The drawing under review shows one solid part. Ordinate dimensions are in mm from its lowest x, y, z. A direction names the side the tool comes from. Give positions to 0.01 mm unless a question says otherwise; leave off trailing zeros. Loops run counter-clockwise (first coordinate to the right, second up) from the corner with the lowest first, then second, coordinate; pieces in that order, holes last.
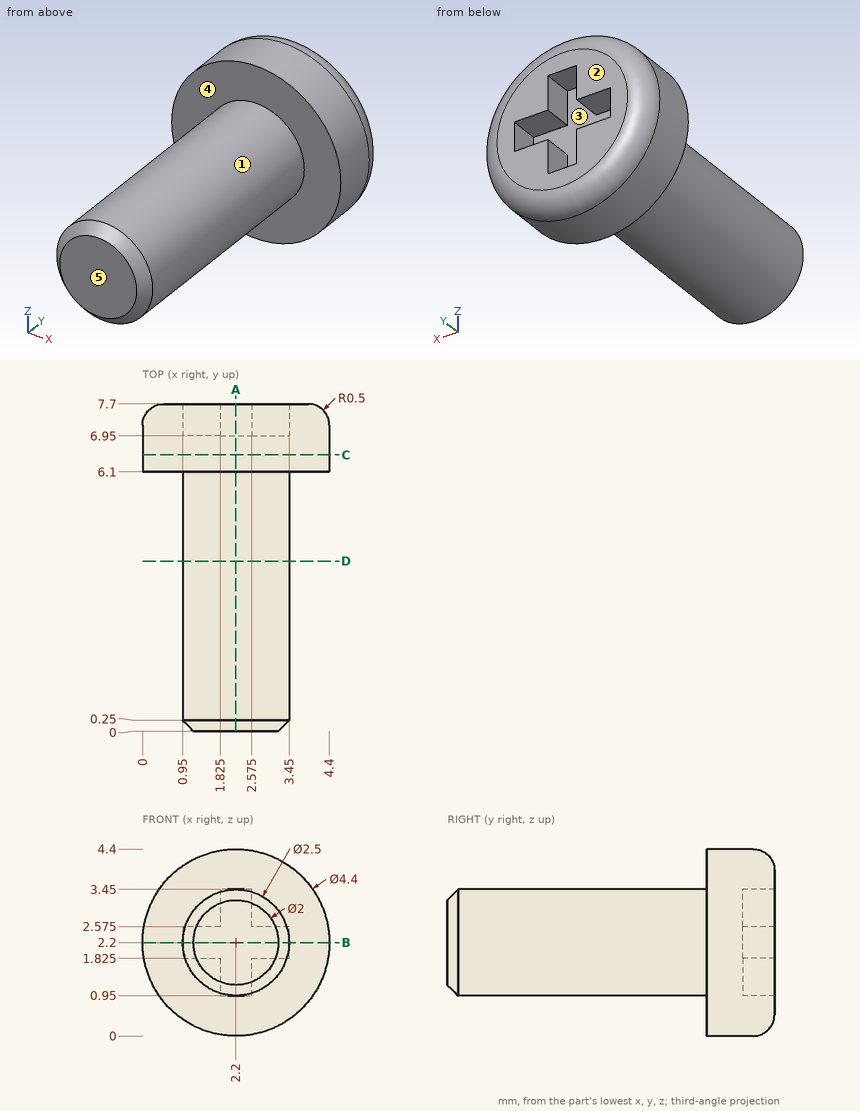
Item 1: Take a section at D-D on y = 4. Give the boundary of the cut face in (x, z).
Answer:
outline: circle Ø2.5 at (2.2, 2.2)
Item 2: Tool access review of the marked faces 4 and 5: name each direction out of +Z, -Z, +X, -X, +Y, -Y from which nothing blocks a thin tool from reaching the whole face with its end or side.
Answer:
face 4: -Y
face 5: +Z, -Z, +X, -X, -Y
Item 3: Take a section at A-A on x = 2.2. Give the boundary of the cut face in (y, z).
Answer:
outline: (0, 1.2) - (0.25, 0.95) - (6.1, 0.95) - (6.1, 0) - (7.2, 0) arc R0.5 ccw to (7.7, 0.5) - (7.7, 0.95) - (6.95, 0.95) - (6.95, 3.45) - (7.7, 3.45) - (7.7, 3.9) arc R0.5 ccw to (7.2, 4.4) - (6.1, 4.4) - (6.1, 3.45) - (0.25, 3.45) - (0, 3.2) - close
Item 4: Take a section at C-C on y = 6.5. Give the boundary of the cut face in (x, z).
Answer:
outline: circle Ø4.4 at (2.2, 2.2)
Item 5: For L1, parallel to Y at x = 3.5, z = 2.1; L2, parallel to Z at x = 1.3, y = 7.25 (3 decimals); L3, parallel to Y at x = 1.7, z = 2.45, list the stretches that pass through material, from the lowest coordinate up.
Answer:
L1: y = 6.1 to 7.7
L2: z = 0.195 to 1.825, 2.575 to 4.205
L3: y = 0 to 6.95
Item 6: The part is to be moulded in two halves that separate along Z. For the marked faces 1, 2 and 3, say which applies: released by +Z, released by -Z, zero draft, split by the parting line, or undercut.
Answer:
face 1: split by the parting line
face 2: zero draft
face 3: undercut
Item 7: Take a section at B-B on z = 2.2. Give the boundary of the cut face in (x, y).
Answer:
outline: (0, 6.1) - (0.95, 6.1) - (0.95, 0.25) - (1.2, 0) - (3.2, 0) - (3.45, 0.25) - (3.45, 6.1) - (4.4, 6.1) - (4.4, 7.2) arc R0.5 ccw to (3.9, 7.7) - (3.45, 7.7) - (3.45, 6.95) - (0.95, 6.95) - (0.95, 7.7) - (0.5, 7.7) arc R0.5 ccw to (0, 7.2) - close
Item 8: Clearance check with flat-ended pins moving along their axes: pin 1 Ø2 at (y, z) = (5, 2) entering from +X; pin 2 Ø2 at (x, y) = (1, 2) entering from +Z; pin 3 Ø0.8 at (x, y) = (3, 7.5) entering from +Z. State where each tip first meets the part, or that it passes through.
Answer:
pin 1: stops at x = 3.45
pin 2: stops at z = 3.43
pin 3: stops at z = 4.34
